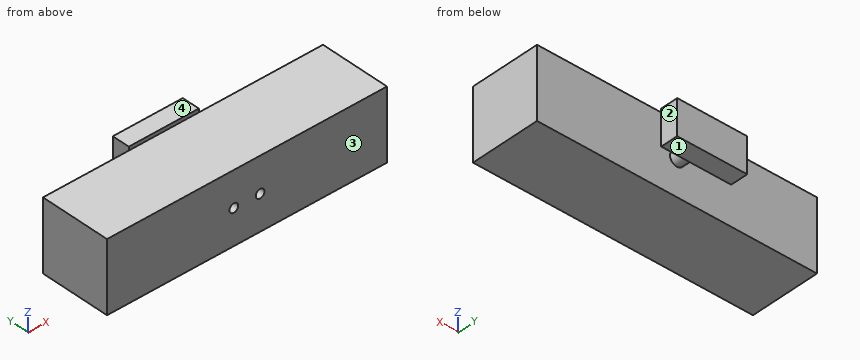
```python
from build123d import *

# Parameters (mm, degrees)
F0_W     = 101.6
F0_H     = 25.4
F0_R     = 1.5875
F1_DEPTH = 25.4
F2_R     = 2.54
F3_DEPTH = 7.62
F4_W     = 25.4
F4_H     = 12.7
F5_DEPTH = 6.35
F6_DEPTH = 19.05


with BuildPart() as f1:
    # F0 (on Front) → F1 (new body)
    with BuildSketch(Plane.XZ):
        Rectangle(F0_W, F0_H)
        with Locations((-4.7625, 0)):
            Circle(F0_R, mode=Mode.SUBTRACT)
        with Locations((4.7625, 0)):
            Circle(F0_R, mode=Mode.SUBTRACT)
        with Locations((4.7625, 0)):
            Circle(F0_R)
        with Locations((-4.7625, 0)):
            Circle(F0_R)
    extrude(amount=-F1_DEPTH)

    # F2 (on face) → F3 (join)
    with BuildSketch(Plane(origin=(0, 25.4, 0), x_dir=(-1, 0, 0), z_dir=(0, 1, 0))):
        Circle(F2_R)
    extrude(amount=F3_DEPTH)

    # F4 (on face) → F5 (join)
    with BuildSketch(Plane(origin=(0, 33.02, 0), x_dir=(-1, 0, 0), z_dir=(0, 1, 0))):
        Rectangle(F4_W, F4_H)
    extrude(amount=F5_DEPTH)

    # F0 (on Front) → F6 (cut)
    with BuildSketch(Plane.XZ):
        with Locations((-4.7625, 0)):
            Circle(F0_R)
        with Locations((4.7625, 0)):
            Circle(F0_R)
    extrude(amount=-F6_DEPTH, mode=Mode.SUBTRACT)


solid = f1.part
```
Part model, mm, in its own coordinate system. Face numbers are marked on the shaded views. A direction names the side the tool comes from. Give positions to 0.01 mm unless a question says otherwise; leave off trailing zeros. Order: outer loops, then holes, each group sorted by start corner. A loop starts at its lowest first (then second) coordinate and runs counter-clockwise, first axis right, second up. Notation, with made-up numbers: M 89.5,-4 L 129.5,-4 A22 ccw 129.5,35 Z; hole C 22,-17 d10. An arc over 180 degrees is marked long. Use a Markdown table: item, result. Add a question column.
(1) 3-axis set-ups, long thin cutter, end or side, ignore diameter. For the marked faces 1, 2, 3 and 4: which of +Z, -Z, +X, -X, +Y, -Y reach the whole face in a straight line?
(2) Saw through at D-D, the plane y = 35.5. Give the cut face in (x, z).
(3) Probe line 1 along Y through (x, z) = (12, -1); line 2 along Y through (x, z) = (-12, -6.75). List the from-to ranges inside material, lowest first. Write a range as [from, to].
(4) Saw through at C-C, the plane x = 0. Give the cut face in (y, z).
(5) Saw through at A-A, the plane z = 5. Give the cut face in (x, y).
(6) Drop flat-ended pins along their axis: P1, Ø1.6, axis at x = 4.5, z = -0.5, coming from the -Y side; P2, Ø6, axis at x = 37, z = 3, coming from the +Y side; P3, Ø5, axis at x = -2, y = 35, coming from the -Z side. Give the stop position or say it passes through.
(7) Saw through at B-B, the plane z = 0. Give the cut face in (x, y) (3 decimals).
Answer key:
| question | item | result |
|---|---|---|
| 1 | face 1 | -Z, +X, -X, +Y |
| 1 | face 2 | +Z, -Z, +X, +Y |
| 1 | face 3 | +Z, -Z, +X, -X, -Y |
| 1 | face 4 | +Z, +X, -X, +Y |
| 2 | outline | M -12.7,-6.35 L 12.7,-6.35 L 12.7,6.35 L -12.7,6.35 Z |
| 3 | line 1 | [0, 25.4], [33.02, 39.37] |
| 3 | line 2 | [0, 25.4] |
| 4 | outline | M 0,-12.7 L 25.4,-12.7 L 25.4,-2.54 L 33.02,-2.54 L 33.02,-6.35 L 39.37,-6.35 L 39.37,6.35 L 33.02,6.35 L 33.02,2.54 L 25.4,2.54 L 25.4,12.7 L 0,12.7 Z |
| 5 | outline | M -50.8,0 L 50.8,0 L 50.8,25.4 L -50.8,25.4 Z; M -12.7,33.02 L 12.7,33.02 L 12.7,39.37 L -12.7,39.37 Z |
| 6 | P1 | y = 19.05 |
| 6 | P2 | y = 25.4 |
| 6 | P3 | z = -6.35 |
| 7 | outline | M -50.8,0 L -6.35,0 L -6.35,19.05 L -3.175,19.05 L -3.175,0 L 3.175,0 L 3.175,19.05 L 6.35,19.05 L 6.35,0 L 50.8,0 L 50.8,25.4 L 2.54,25.4 L 2.54,33.02 L 12.7,33.02 L 12.7,39.37 L -12.7,39.37 L -12.7,33.02 L -2.54,33.02 L -2.54,25.4 L -50.8,25.4 Z |
